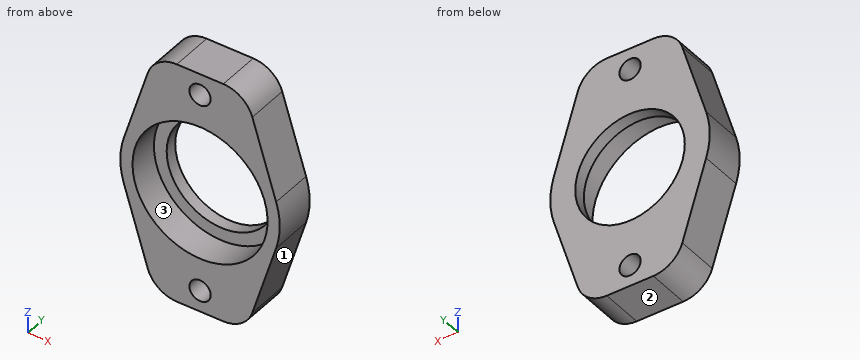
Autodesk Inventor part; units mm, degrees
ref_plane "YZ Plane" through (0, 0, 0) normal (1, 0, 0) x (0, 1, 0)
ref_plane "XZ Plane" through (0, 0, 0) normal (0, 1, 0) x (-1, 0, 0)
ref_plane "XY Plane" through (0, 0, 0) normal (0, 0, 1) x (1, 0, 0)
sketch "Szkic1" plane through (0, 0, 0) normal (0, 1, 0) x (-1, 0, 0)
  circle A0 centre (0, 0) radius 11.1
  circle A1 centre (0, 0) radius 13.1
  line L0 (-7.5, 20) -> (7.5, 20)
  line L1 (0, 20) -> (0, 0) construction
  line L2 (7.5, 20) -> (12.5093, 3.8895)
  line L3 (-7.5, 20) -> (-12.5093, 3.8895)
  circle A2 centre (0, 16.5) radius 1.75
  line L4 (0, 0) -> (13.1, 0) construction
  line L5 (-7.5, -20) -> (7.5, -20)
  line L6 (0, -20) -> (0, 0) construction
  line L7 (7.5, -20) -> (12.5093, -3.8895)
  line L8 (-7.5, -20) -> (-12.5093, -3.8895)
  circle A3 centre (0, -16.5) radius 1.75
  arc A4 (12.5093, 3.8895) -> (-12.5093, 3.8895) centre (0, 0) ccw
  arc A5 (-12.5093, -3.8895) -> (12.5093, -3.8895) centre (0, 0) ccw
  dimension "d0" = 22.2
  dimension "d1" = 2
  dimension "d2" = 15
  dimension "d3" = 20
  dimension "d7" = 16.5
  dimension "d8" = 3.5
extrude "Wyciągnięcie proste1" add sketch "Szkic1" along normal blind 7
sketch "Szkic2" plane through (0, 7, 0) normal (0, 1, 0) x (1, 0, 0)
  circle A0 centre (0, 0) radius 13.1
  arc A1 (-12.5093, 3.8895) -> (-12.5093, -3.8895) centre (0, 0) ccw construction
  circle A2 centre (0, 0) radius 9
  circle A3 centre (0, 0) radius 11.1 construction
  dimension "d22" = 18
extrude "Wyciągnięcie proste2" add sketch "Szkic2" against normal blind 2
fillet "Zaokrąglenie1" radius 5 4 edges at (-7.5, 3.5, 20) (7.5, 3.5, 20) (7.5, 3.5, -20) (-7.5, 3.5, -20)
properties part number "CH_01_0022_bearing_mount"
For this review, take the finished solid that the model builds, in its own axes (mm). Face numbers are marked on the shaded views. Round coordinates to 2 decimals unless told otherwise and drop trailing zeros. Write each loop counter-clockwise with the first axis right and the second up, starting at its lowest first coordinate (ties: lowest second). Pieces come first, ordered by that corner, then holes. Notation, with made-up numbers: (46, 78) -> (77, 78) arc R18 cw to (77, 102) -> close; hole circle Ø11 at (4, 34.25). An arc over 180 degrees is marked (long way). One line per question, with ' | ' between items. Start each with the question number.
1) Add section C-C (y = 5.75). Write out the cut boundary in (x, z), and give its area (3 significant figures).
2) Wall thickness on line 1 along Z through (x, y) = (0, 1.2); line 2 along Z through (x, y) = (0, 6.5); line 3 along X through (y, z) = (5.9, 0): over which ranges is each line inside the solid? List them lowest first.
3) Add section D-D (x = 6). Write out the cut boundary in (y, z).
4) Add section B-B (z = 0). Write out the cut boundary in (x, y).
5) For pin 1 Ø1 at (y, z) = (3.5, -10.5) entering from +X; pin 2 Ø3 at (x, z) = (0, -16.5) entering from -Y; pin 3 Ø1.5 at (y, z) = (1.5, -7) entering from -X; pin 4 Ø4 at (y, z) = (2.5, 13) entering from -X, all flat-tipped, find the tip position at first contact; note any pin that passes through.
6) Add section A-A (x = 0). Write out the cut boundary in (y, z).
7) Mouldability with a two-part tool opening along X and no side actions: class the marked faces 1, 2 and 3 as +X half, -X half, draft (parallel to the pull), parting line (faces both ways), or undercut.
Reported:
1) outline: (-12.51, -3.89) -> (-8.59, -16.48) arc R5 ccw to (-3.82, -20) -> (3.82, -20) arc R5 ccw to (8.59, -16.48) -> (12.51, -3.89) arc R13.1 ccw to (12.51, 3.89) -> (8.59, 16.48) arc R5 ccw to (3.82, 20) -> (-3.82, 20) arc R5 ccw to (-8.59, 16.48) -> (-12.51, 3.89) arc R13.1 ccw to start; hole circle Ø18 at (0, 0); hole circle Ø3.5 at (0, -16.5); hole circle Ø3.5 at (0, 16.5) | area: 562 mm²
2) line 1: z = -20 to -18.25, -14.75 to -11.1, 11.1 to 14.75, 18.25 to 20 | line 2: z = -20 to -18.25, -14.75 to -9, 9 to 14.75, 18.25 to 20 | line 3: x = -13.1 to -9, 9 to 13.1
3) outline: (0, -19.5) -> (7, -19.5) -> (7, -6.71) -> (5, -6.71) -> (5, -9.34) -> (0, -9.34) -> close; (0, 9.34) -> (5, 9.34) -> (5, 6.71) -> (7, 6.71) -> (7, 19.5) -> (0, 19.5) -> close
4) outline: (-13.1, 0) -> (-11.1, 0) -> (-11.1, 5) -> (-9, 5) -> (-9, 7) -> (-13.1, 7) -> close; (9, 5) -> (11.1, 5) -> (11.1, 0) -> (13.1, 0) -> (13.1, 7) -> (9, 7) -> close
5) pin 1: stops at x = 10.61 | pin 2: passes through | pin 3: stops at x = -11.78 | pin 4: stops at x = -10.3
6) outline: (0, -20) -> (7, -20) -> (7, -18.25) -> (0, -18.25) -> close; (0, -14.75) -> (7, -14.75) -> (7, -9) -> (5, -9) -> (5, -11.1) -> (0, -11.1) -> close; (0, 11.1) -> (5, 11.1) -> (5, 9) -> (7, 9) -> (7, 14.75) -> (0, 14.75) -> close; (0, 18.25) -> (7, 18.25) -> (7, 20) -> (0, 20) -> close
7) face 1: +X half | face 2: draft | face 3: undercut
